Answer from the drawing. Dimensions are ordinates in mm from the lowest x, y and z of the part. A direction names the side the tool comes from. Give positions to 0.01 mm unless a question says otherwise; leave off trailing zeros. Loops run counter-clockwise (first coordinate to the right, second up) from the corner with the lowest first, then second, coordinate; pieces in that order, holes last. Notation, with made-up numbers: (35.5, 7.5) - (94.5, 7.5) arc R15 ccw to (94.5, 23.5) - close; hole circle Ø11 at (78, -0.75). An arc over 180 degrees is marked (long way). Put each result on its own line as item: value. Start each with the question number.
1. A cutting plane is placed at B-B, the plane y = 36. Determine the outline of the cut face in (x, z).
2. A cutting plane is placed at A-A, the plane z = 25. Determine the outline of the cut face in (x, y).
3. For the marked faces 1, 2 and 3, determine the directions among +Z, -Z, +X, -X, +Y, -Y from which every point of the face is accessible in a straight line to the end or side of a thin tool.
4. Given pin 1 Ø5 at (x, y) = (37, 10.5) entering from +Z; pin 2 Ø4 at (x, z) = (51.8, 61.41) entering from +Y; pin 3 Ø5 at (y, z) = (20, 39.5) entering from -X; pin 4 Ø1.5 at (x, y) = (51.5, 31.5) entering from +Z, each flat-ended and moving along its own axis, determine where each tip first touches the part or whether it passes through.
5. A cutting plane is placed at C-C, the plane x = 3.2. Determine the outline of the cut face in (y, z), plus the area to 3 significant figures.
6. For a pull along Y with two mould halves and no side action, classify the marked faces 4, 5, 6 and 7 as released by +Y, released by -Y, zero draft, split by the parting line, or undercut.
7. Consider L1, parallel to Z at x = 51.8, y = 31.75; L2, parallel to Z at x = 46.5, y = 42; L3, parallel to Y at x = 50.5, z = 63. Determine where each line is inside the solid, lowest interval first. Write a range as from..to.
8. A cutting plane is placed at D-D, the plane x = 40.5. Determine the outline of the cut face in (y, z).
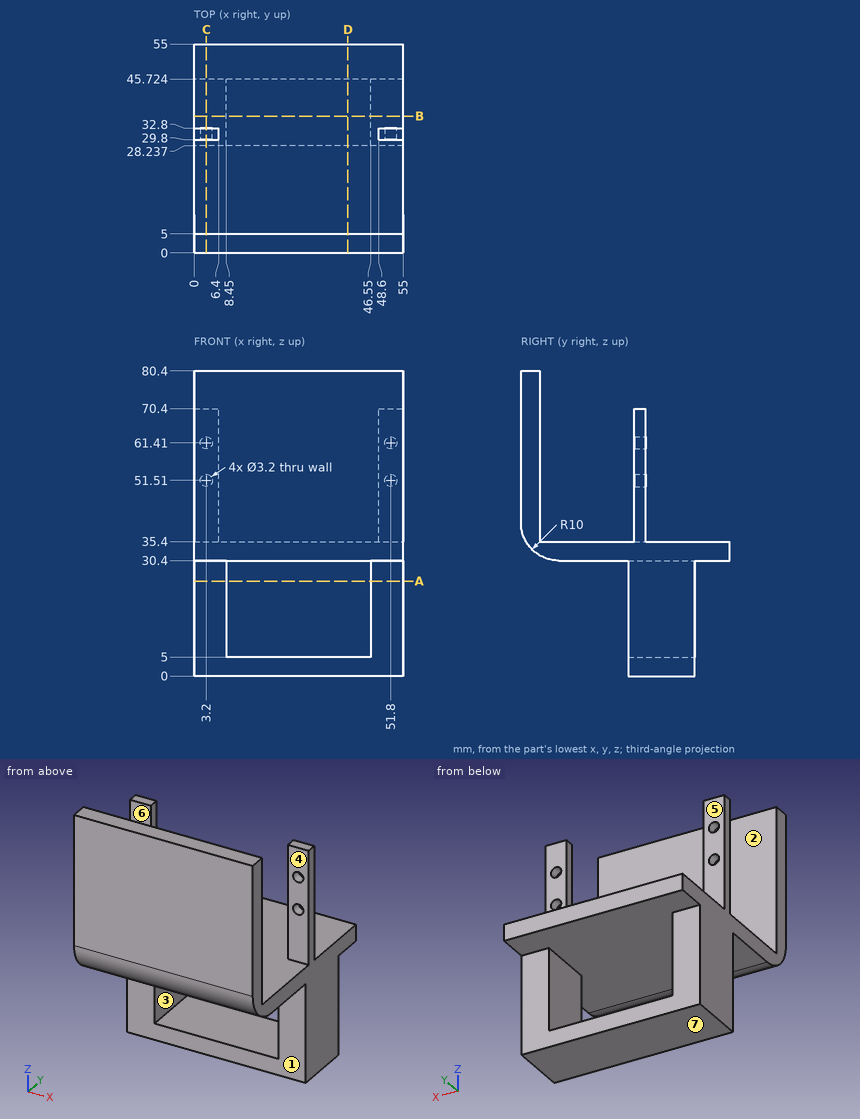
Return value:
1. outline: (0, 0) - (55, 0) - (55, 35.4) - (0, 35.4) - close; hole (8.45, 5) - (46.55, 5) - (46.55, 30.4) - (8.45, 30.4) - close
2. outline: (0, 28.24) - (8.45, 28.24) - (8.45, 45.72) - (0, 45.72) - close; (46.55, 28.24) - (55, 28.24) - (55, 45.72) - (46.55, 45.72) - close
3. face 1: -Z, +X, -X, -Y
3. face 2: +Z, +X, -X
3. face 3: +Y, -Y
4. pin 1: stops at z = 35.4
4. pin 2: stops at y = 32.8
4. pin 3: passes through
4. pin 4: stops at z = 70.4
5. outline: (0, 40.4) arc R10 ccw to (10, 30.4) - (28.24, 30.4) - (28.24, 0) - (45.72, 0) - (45.72, 30.4) - (55, 30.4) - (55, 35.4) - (32.8, 35.4) - (32.8, 49.91) - (29.8, 49.91) - (29.8, 35.4) - (5, 35.4) - (5, 80.4) - (0, 80.4) - close; (29.8, 53.11) - (32.8, 53.11) - (32.8, 59.81) - (29.8, 59.81) - close; (29.8, 63.01) - (32.8, 63.01) - (32.8, 70.4) - (29.8, 70.4) - close
5. area: 1,100 mm2
6. face 4: undercut
6. face 5: released by +Y
6. face 6: undercut
6. face 7: zero draft
7. L1: z = 0..49.91, 53.11..59.81, 63.01..70.4
7. L2: z = 0..5, 30.4..35.4
7. L3: y = 0..5, 29.8..32.8
8. outline: (0, 40.4) arc R10 ccw to (10, 30.4) - (55, 30.4) - (55, 35.4) - (5, 35.4) - (5, 80.4) - (0, 80.4) - close; (28.24, 0) - (45.72, 0) - (45.72, 5) - (28.24, 5) - close
